Check sheet for the modelled part. Datum: model origin and axes. Units: mm. Round coordinates to 2 decimals unless told otherwise and drop trailing zeros. Loops run counter-clockwise (first coordinate to the right, second up) from the corner with the lowest first, then second, coordinate; pieces in that order, holes last. Notation, with made-up numbers: (87.25, 49) -> (99.25, 49) arc R28 cw to (99.25, 87) -> close; hole circle Ø6 at (73.25, 77). An arc over 180 degrees is marked (long way). One line per item, written item: value. Start each with the question number.
1. Cross-section at A-A on x = -76.5. Record the cut outline in (y, z).
2. Cross-section at D-D on z = -33. Record the cut outline in (x, y), then the cut area to 3 significant figures.
3. Material ranges on L1, parallel to X at y = 2.25, z = -6; L2, parallel to X at y = 5.5, z = 33; L3, parallel to X at y = 2, z = 200, recorded low to high.
4. Cross-section at C-C on z = 1. Record the cut outline in (x, y).
5. Go/stop test with flat-tipped pins: pin 1 (3 mm diameter, centred on y = 2.5, z = 0, fed in from +X); pin 2 (3 mm diameter, centred on y = 3, z = -22.5, fed in from -X). Record where each tip stops, or that it passes through.
6. Cross-section at B-B on z = 199. Record the cut outline in (x, y).
from build123d import *

# Parameters (mm, degrees)
BOSS_EXTRUDE1_DEPTH = 6.35
SKETCH2_W           = 12.7
SKETCH2_H           = 76.2
SKETCH2_W_2         = 76.2
SKETCH2_H_2         = 12.7
SKETCH2_W_3         = 25.4
SKETCH2_H_3         = 88.9
CUT_EXTRUDE1_DEPTH  = 286.467638271
SKETCH3_W           = 12.7
SKETCH3_H           = 50.8
CUT_EXTRUDE2_DEPTH  = 286.467638271


with BuildPart() as part:
    # Sketch1 → Boss-Extrude1 (new body)
    with BuildSketch(Plane(origin=(0, 0, 0), x_dir=(1, 0, 0), z_dir=(0, 1, 0))):
        Polygon((-152.4, 76.2), (-152.4, -241.3), (-44.45, -241.3), (-44.45, -76.2), (44.45, -76.2), (44.45, -241.3), (152.4, -241.3), (152.4, 76.2), align=None)
    extrude(amount=BOSS_EXTRUDE1_DEPTH)

    # Sketch2 → Cut-Extrude1 (cut, through all)
    with BuildSketch(Plane(origin=(0, 6.35, 0), x_dir=(1, 0, 0), z_dir=(0, 1, 0))):
        with Locations((146.05, 1.27)):
            Rectangle(SKETCH2_W, SKETCH2_H)
        with Locations((146.05, -177.8)):
            Rectangle(SKETCH2_W, SKETCH2_H)
        with Locations((-146.05, -177.8)):
            Rectangle(SKETCH2_W, SKETCH2_H)
        with Locations((-146.05, 1.27)):
            Rectangle(SKETCH2_W, SKETCH2_H)
        with Locations((-76.2, 69.85)):
            Rectangle(SKETCH2_W_2, SKETCH2_H_2)
        with Locations((76.2, 69.85)):
            Rectangle(SKETCH2_W_2, SKETCH2_H_2)
        with Locations((-76.2, 6.35)):
            Rectangle(SKETCH2_W_3, SKETCH2_H_3)
        with Locations((76.2, 6.35)):
            Rectangle(SKETCH2_W_3, SKETCH2_H_3)
    extrude(amount=-CUT_EXTRUDE1_DEPTH, mode=Mode.SUBTRACT)

    # Sketch3 → Cut-Extrude2 (cut, through all)
    with BuildSketch(Plane(origin=(0, 6.35, 0), x_dir=(1, 0, 0), z_dir=(0, 1, 0))):
        with Locations((-38.1, 0)):
            Rectangle(SKETCH3_W, SKETCH3_H)
        with Locations((38.1, 0)):
            Rectangle(SKETCH3_W, SKETCH3_H)
    extrude(amount=-CUT_EXTRUDE2_DEPTH, mode=Mode.SUBTRACT)


solid = part.part
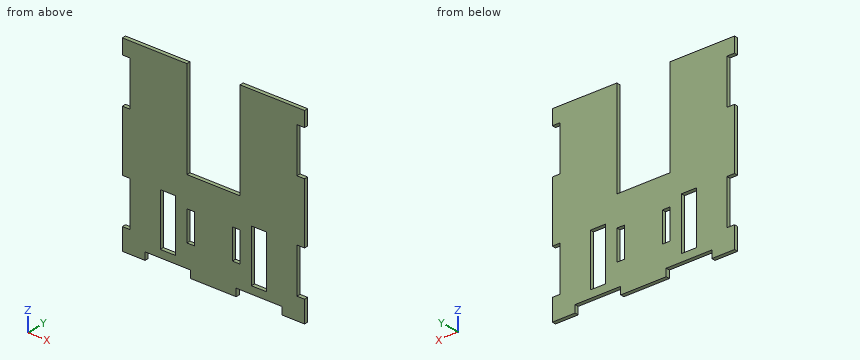
Taken from the geometry:
1. outline: (0, -63.5) -> (6.35, -63.5) -> (6.35, -50.8) -> (0, -50.8) -> close; (0, 38.1) -> (6.35, 38.1) -> (6.35, 241.3) -> (0, 241.3) -> close
2. outline: (-139.7, 0) -> (-88.9, 0) -> (-88.9, 6.35) -> (-139.7, 6.35) -> close; (-63.5, 0) -> (63.5, 0) -> (63.5, 6.35) -> (-63.5, 6.35) -> close; (88.9, 0) -> (139.7, 0) -> (139.7, 6.35) -> (88.9, 6.35) -> close
2. area: 1,450 mm2
3. L1: x = -139.7 to -88.9, -63.5 to -44.45, -31.75 to 31.75, 44.45 to 63.5, 88.9 to 139.7
3. L2: x = -139.7 to -88.9, -63.5 to 63.5, 88.9 to 139.7
3. L3: x = -139.7 to -44.45, 44.45 to 139.7
4. outline: (-139.7, 0) -> (-88.9, 0) -> (-88.9, 6.35) -> (-139.7, 6.35) -> close; (-63.5, 0) -> (-44.45, 0) -> (-44.45, 6.35) -> (-63.5, 6.35) -> close; (-31.75, 0) -> (31.75, 0) -> (31.75, 6.35) -> (-31.75, 6.35) -> close; (44.45, 0) -> (63.5, 0) -> (63.5, 6.35) -> (44.45, 6.35) -> close; (88.9, 0) -> (139.7, 0) -> (139.7, 6.35) -> (88.9, 6.35) -> close
5. pin 1: stops at x = 139.7
5. pin 2: stops at x = -139.7
6. outline: (-139.7, 0) -> (-44.45, 0) -> (-44.45, 6.35) -> (-139.7, 6.35) -> close; (44.45, 0) -> (139.7, 0) -> (139.7, 6.35) -> (44.45, 6.35) -> close
